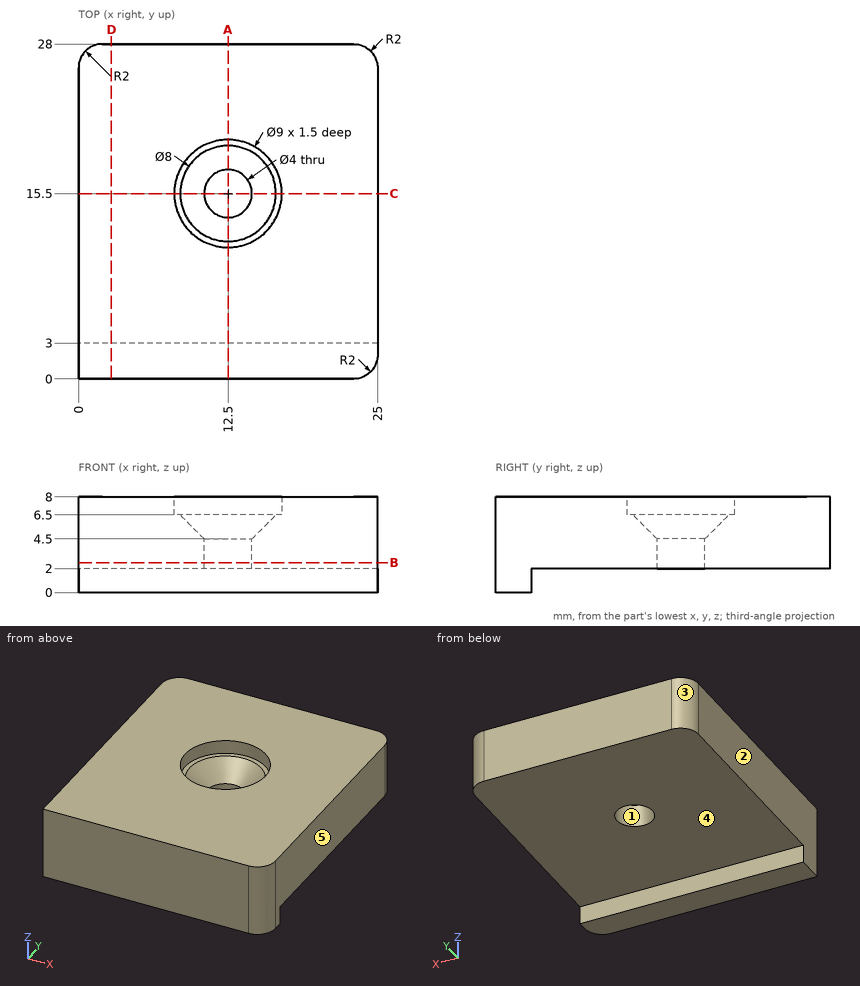
Could you check a few things on this drawing? It's one solid part, dimensions in mm from its lowest x, y, z. A direction names the side the tool comes from. Coordinates: 2 decimals unless noted, no trailing zeros. Loops run counter-clockwise (first coordinate to the right, second up) from the corner with the lowest first, then second, coordinate; pieces in that order, holes last.
1. For P1, Ø2.5, axis at x = 10.5, y = 15.5, coming from the +Z side; P2, Ø12.5, axis at x = 7.5, y = 19.5, coming from the -Z side; P3, Ø0.6, axis at x = 12.5, z = 1, coming from the +Y side, each with a flat end and sliding along its axis, tell me the tip position at first contact or that it passes through.
2. Imagine slicing it at D-D (x = 2.75). Please give me the cut outline in (y, z), and give its area (3 significant figures).
3. We'd pull the mould along Y, two halves only. Please class the marked faces 1, 2 and 3: released by +Y, released by -Y, zero draft, split by the parting line, or undercut.
4. Imagine slicing it at C-C (y = 15.5). Please give me the cut outline in (x, z), and give its area (4 significant figures).
5. Imagine slicing it at A-A (x = 12.5). Please give me the cut outline in (y, z), and give its area (4 significant figures).
6. Imagine slicing it at B-B (z = 2.5). Please give me the cut outline in (x, y), and give its area (3 significant figures).
7. For the marked faces 4 and 5, which set-ups out of +Z, -Z, +X, -X, +Y, -Y let a thin tool reach every point of the face, with its end or its side?
8. I need wall thicknesses on L1, parallel to Y at x = 12.5, z = 7.6; L2, parallel to Z at x = 22, y = 15.5; L3, parallel to Y at x = 11.25, z = 7. Which ranges of each line are inside material? Lowest first, please.
Computed values:
1. P1: stops at z = 5.75
1. P2: stops at z = 2
1. P3: stops at y = 3
2. outline: (0, 0) - (3, 0) - (3, 2) - (28, 2) - (28, 8) - (0, 8) - close
2. area: 174 mm2
3. face 1: undercut
3. face 2: zero draft
3. face 3: released by +Y
4. outline: (0, 2) - (10.5, 2) - (10.5, 4.5) - (8.5, 6.5) - (8, 6.5) - (8, 8) - (0, 8) - close; (14.5, 2) - (25, 2) - (25, 8) - (17, 8) - (17, 6.5) - (16.5, 6.5) - (14.5, 4.5) - close
4. area: 114.5 mm2
5. outline: (0, 0) - (3, 0) - (3, 2) - (13.5, 2) - (13.5, 4.5) - (11.5, 6.5) - (11, 6.5) - (11, 8) - (0, 8) - close; (17.5, 2) - (28, 2) - (28, 8) - (20, 8) - (20, 6.5) - (19.5, 6.5) - (17.5, 4.5) - close
5. area: 138.5 mm2
6. outline: (0, 0) - (23, 0) arc R2 ccw to (25, 2) - (25, 26) arc R2 ccw to (23, 28) - (2, 28) arc R2 ccw to (0, 26) - close; hole circle Ø4 at (12.5, 15.5)
6. area: 685 mm2
7. face 4: -Z, +X, -X, +Y
7. face 5: +Z, -Z, +X, +Y, -Y
8. L1: y = 0 to 11, 20 to 28
8. L2: z = 2 to 8
8. L3: y = 0 to 11.18, 19.82 to 28
